Model file for the job. Use its own axes, mm. Face numbers are marked on the shaded views. A direction names the side the tool comes from. Round coordinates to 2 decimals unless told otherwise and drop trailing zeros. Loops run counter-clockwise (first coordinate to the right, second up) from the corner with the lowest first, then second, coordinate; pieces in that order, holes last. Notation, with made-up numbers: M 14,76.25 L 42,76.25 A24 cw 42,87.25 Z; hole C 80.25,14.25 d6. An arc over 180 degrees is marked long. Use a Markdown table: item, result. Add a question column.
Item 1: Saw through at C-C on z = -12.7. Write the cut outline in (x, y) (1 decimal).
Item 2: Wall check: L1, parallel to Z at x = 0, y = 2.25 (1 decimal); L2, parallel to X at y = 1.45, z = 0 (1 decimal); L3, parallel to Z at x = 0, y = 4.25. Give the ranges that are in metal, low to high. Write a range as from..to.
Item 3: Pin check, flat tips, straight feed: P1, Ø1, axis at y = 5.5, z = -5, coming from the +X side; P2, Ø3.5, axis at x = 0, y = 6.35, coming from the +Z side; P3, Ø1.5, axis at y = 1.5, z = -5, coming from the +X side. Stop position of each tip, or through.
Item 4: Tool access for the marked faces 5 and 6: list every direction of +Z, -Z, +X, -X, +Y, -Y with a clear straight run to the whole face (end or side of a thin tool).
Item 5: Two-plate mould, pull along X, no slides. Class the marked faces 1, 2, 3 and 4: +X half, -X half, draft (parallel to the pull), parting line (faces both ways), or undercut.
Item 6: Saw through at B-B on x = 12.7. Write the cut outline in (y, z) (1 decimal), then the cut area to 3 significant figures.
Item 7: Saw through at A-A on z = 0. Give the number of separate pieces and of enclosed holes in the cut face, then the cut area to 3 significant figures.
Item 8: Saw through at D-D on x = 3. Write the cut outline in (y, z) (3 decimals), then the cut area to 3 significant figures.
```python
from build123d import *

# Parameters (mm, degrees)
SKETCH1_R           = 15.875
SKETCH1_R_2         = 1.5875
BOSS_EXTRUDE1_DEPTH = 3.175
SKETCH2_R           = 6.35
BOSS_EXTRUDE2_DEPTH = 6.35
SKETCH3_R           = 1.5875
CUT_EXTRUDE1_DEPTH  = 10.525


with BuildPart() as part:
    # Sketch1 → Boss-Extrude1 (new body)
    with BuildSketch(Plane(origin=(0, 0, 0), x_dir=(1, 0, 0), z_dir=(0, 1, 0))):
        Circle(SKETCH1_R)
        with Locations((0, 12.7)):
            Circle(SKETCH1_R_2, mode=Mode.SUBTRACT)
        with Locations((12.7, 0)):
            Circle(SKETCH1_R_2, mode=Mode.SUBTRACT)
    extrude(amount=BOSS_EXTRUDE1_DEPTH)

    # Sketch2 → Boss-Extrude2 (add)
    with BuildSketch(Plane(origin=(0, 3.175, 0), x_dir=(1, 0, 0), z_dir=(0, 1, 0))):
        Circle(SKETCH2_R)
    extrude(amount=BOSS_EXTRUDE2_DEPTH)

    # Sketch3 → Cut-Extrude1 (cut, through all)
    with BuildSketch(Plane(origin=(0, 9.525, 0), x_dir=(1, 0, 0), z_dir=(0, 1, 0))):
        Circle(SKETCH3_R)
    extrude(amount=-CUT_EXTRUDE1_DEPTH, mode=Mode.SUBTRACT)

    # Sketch5 → #38 (0.1015) Diameter Hole1 (revolve, cut)
    with BuildSketch(Plane(origin=(0, 6.35, 0), x_dir=(0, 1, 0), z_dir=(1, 0, 0))):
        Polygon((0, 0), (0, 26.174539381), (1.28905, 25.4), (1.28905, 0), align=None)
    revolve(axis=Axis((0, 6.35, -6.35), (0, 0, 1)), mode=Mode.SUBTRACT)


solid = part.part
```
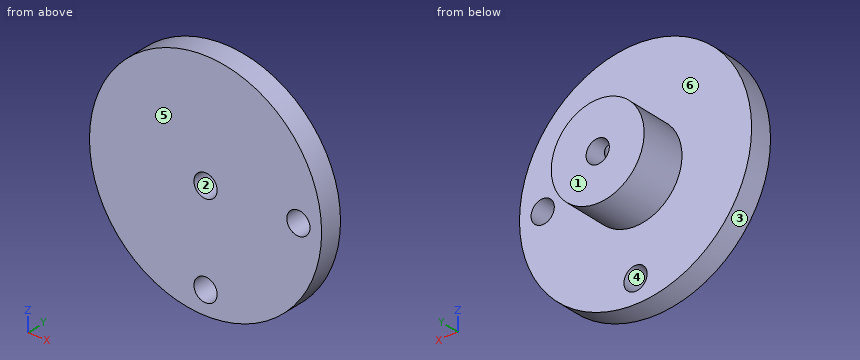
Entries:
| question | item | result |
|---|---|---|
| 1 | outline | M -9.5,0 L -1.6,0 L -1.6,3.2 L -9.5,3.2 Z; M 1.6,0 L 9.5,0 L 9.5,3.2 L 1.6,3.2 Z |
| 2 | L1 | -15.9..-14.3, -11.1..-1.6, 1.6..15.9 |
| 2 | L2 | -15.9..-1.6, 1.6..11.1, 14.3..15.9 |
| 2 | L3 | -6.35..-1.59, 1.59..6.35 |
| 3 | P1 | x = 4.48 |
| 3 | P2 | z = 6.35 |
| 3 | P3 | x = 15.3 |
| 4 | face 5 | +Z, -Z, +X, -X, -Y |
| 4 | face 6 | +Y |
| 5 | face 1 | draft |
| 5 | face 2 | undercut |
| 5 | face 3 | parting line |
| 5 | face 4 | undercut |
| 6 | outline | M 0,-9.5 L 3.2,-9.5 L 3.2,-1.6 L 0,-1.6 Z; M 0,1.6 L 3.2,1.6 L 3.2,9.5 L 0,9.5 Z |
| 6 | area | 50.4 mm2 |
| 7 | separate pieces | 3 |
| 7 | enclosed holes | 0 |
| 7 | area | 141 mm2 |
| 8 | outline | M 0,-15.589 L 3.175,-15.589 L 3.175,-5.597 L 9.525,-5.597 L 9.525,5.597 L 3.175,5.597 L 3.175,15.589 L 0,15.589 Z |
| 8 | area | 170 mm2 |
